Check sheet for the drawn part. Datum: minimum x, y, z corner. Units: mm. A direction names the side the tool comes from. Coordinates: 2 decimals unless noted, no trailing zeros. Order: outer loops, then holes, each group sorted by start corner. A loop starts at its lowest first (then second) coordinate and runs counter-clockwise, first axis right, second up.
Q1. Draft check along Y on the marked faces 1, 2, 3 and 4. Enter one of: pulls with the +Y half, pulls with the -Y half, needs draft (parallel to the pull), parting line crosses it, or undercut.
Q2. Cross-section at C-C, the plane z = 7.5. Record the boundary of the cut face in (x, y).
Q3. Cross-section at B-B, the plane y = 10. Record the boundary of the cut face in (x, z), and give its area (3 significant figures).
Q4. Cross-section at A-A, the plane z = 22. Record the boundary of the cut face in (x, y).
Q5. Thickness scan on line 1 (Y direction, x = 86, z = 22); line 2 (Y direction, x = 59, z = 18.75); line 3 (X direction, y = 80, z = 9.5). Record the ranges inside material, lowest first.
Q6. Cross-section at D-D, the plane y = 29.5. Record the boundary of the cut face in (x, z).
Q7. Set-up check for the marked faces 5, 6 and 7: record each of +Z, -Z, +X, -X, +Y, -Y from which the full face is reachable in a straight line by a thin tool's end or side.
Q8. Depth check by flat-ended pin: P1, Ø3, axis at x = 27, z = 5.5, coming from the +Y side; P2, Ø11, axis at y = 79, z = 3.5, coming from the +X side; P3, Ø3, axis at y = 34, z = 6, coming from the -X side. Enter the tip coordinate at first touch or a pass-through.
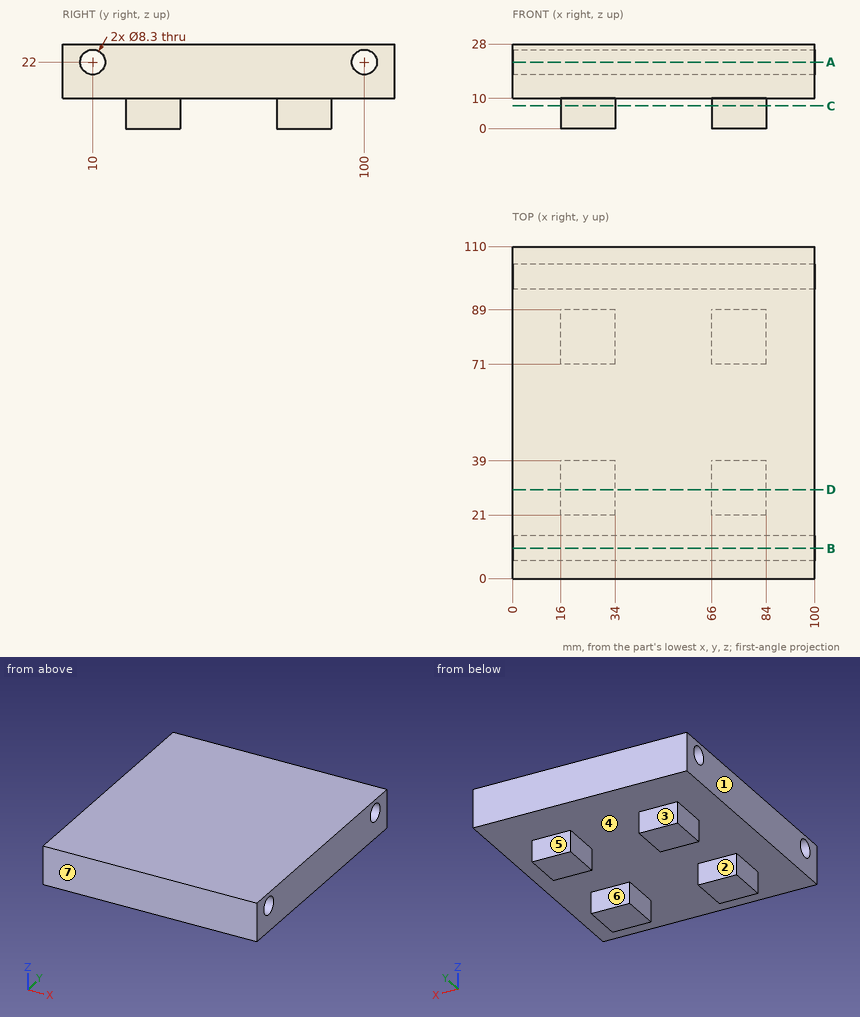
Check values:
1. face 1: needs draft
1. face 2: undercut
1. face 3: pulls with the +Y half
1. face 4: undercut
2. outline: (16, 21) - (34, 21) - (34, 39) - (16, 39) - close; (16, 71) - (34, 71) - (34, 89) - (16, 89) - close; (66, 21) - (84, 21) - (84, 39) - (66, 39) - close; (66, 71) - (84, 71) - (84, 89) - (66, 89) - close
3. outline: (0, 10) - (100, 10) - (100, 17.85) - (0, 17.85) - close; (0, 26.15) - (100, 26.15) - (100, 28) - (0, 28) - close
3. area: 970 mm2
4. outline: (0, 0) - (100, 0) - (100, 5.85) - (0, 5.85) - close; (0, 14.15) - (100, 14.15) - (100, 95.85) - (0, 95.85) - close; (0, 104.15) - (100, 104.15) - (100, 110) - (0, 110) - close
5. line 1: y = 0 to 5.85, 14.15 to 95.85, 104.15 to 110
5. line 2: y = 0 to 7.42, 12.58 to 97.42, 102.58 to 110
5. line 3: x = 16 to 34, 66 to 84
6. outline: (0, 10) - (16, 10) - (16, 0) - (34, 0) - (34, 10) - (66, 10) - (66, 0) - (84, 0) - (84, 10) - (100, 10) - (100, 28) - (0, 28) - close
7. face 5: -Z, +X, -X, +Y
7. face 6: -Z, +X, -X
7. face 7: +Z, -Z, +X, -X, -Y
8. P1: stops at y = 89
8. P2: stops at x = 84
8. P3: stops at x = 16
